from build123d import *

# Parameters (mm, degrees)
F1_DEPTH = 63.5
F0_W     = 25.755785
F0_H     = 19.05
F2_DEPTH = 25.4
F3_DEPTH = 7.9375
F4_R     = 6.35


with BuildPart() as f1:
    # F0 (on Front) → F1 (new body, symmetric)
    with BuildSketch(Plane.XZ):
        Polygon((41.275, -9.525), (41.275, 9.525), (22.225, 9.525), (-41.275, 9.525), (-41.275, -9.525), align=None)
    extrude(amount=F1_DEPTH, both=True)

    # F0 (on Front) → F2 (join, symmetric)
    with BuildSketch(Plane.XZ):
        with BuildLine():
            Line((22.225, 9.525), (41.275, 9.525))
            Line((41.275, 9.525), (41.275, 34.925))
            ThreePointArc((41.275, 34.925), (45.92468, 46.15032), (57.15, 50.8))
            Line((57.15, 50.8), (60.325, 50.8))
            Line((60.325, 50.8), (60.325, 69.85))
            Line((60.325, 69.85), (57.15, 69.85))
            ThreePointArc((57.15, 69.85), (32.454296, 59.620704), (22.225, 34.925))
            Line((22.225, 34.925), (22.225, 9.525))
        make_face()
        with Locations((73.202892, 60.325)):
            Rectangle(F0_W, F0_H)
    extrude(amount=F2_DEPTH, both=True)

    # F0 (on Front) → F3 (join, symmetric)
    with BuildSketch(Plane.XZ):
        with BuildLine():
            Line((-41.275, 9.525), (22.225, 9.525))
            Line((22.225, 9.525), (22.225, 34.925))
            ThreePointArc((22.225, 34.925), (32.454296, 59.620704), (57.15, 69.85))
            add(Edge.make_bspline(
                [(-41.275, 9.525), (-27.324263, 47.769934), (18.911634, 71.788173), (57.15, 69.85)],
                knots=[0, 0, 0, 0, 115.440834, 115.440834, 115.440834, 115.440834], degree=3))
        make_face()
    extrude(amount=F3_DEPTH, both=True)

    # F4
    f4_edges = [f1.edges().sort_by_distance(p)[0] for p in [
        (41.275, -63.5, 0),
        (-41.275, -63.5, 0),
        (41.275, 63.5, 0),
        (-41.275, 63.5, 0),
    ]]
    fillet(f4_edges, radius=F4_R)


solid = f1.part
Could you check a few things on this model? Use its own coordinates, in mm. A direction names the side the tool comes from. Give positions to 0.01 mm unless a question says otherwise; leave off trailing zeros. Order: outer loops, then holes, each group sorted by start corner. A loop starts at its lowest first (then second) coordinate and runs counter-clockwise, first axis right, second up.
1. Will these pins go through, and if not, where does the flat tip stop? P1, Ø16.5, axis at x = -8, y = -49.5, coming from the +Z side (3 decimals); P2, Ø22, axis at y = -28, z = 15, coming from the +X side (3 decimals); P3, Ø14.5, axis at x = 70.5, y = -5, coming from the -Z side.
2. For faces 1 (the cylindrical face through (32.727, -16.791, 59.891)), 2 (the flat face through (47, -25.4, 54)), 3 (the cylindrical face through (32.727, 16.547, 59.891)), 4 (the flat face through (71, 0, 50.8)), which set-ups out of +Z, -Z, +X, -X, +Y, -Y let a thin tool reach every point of the face, with its end or its side?
3. Suppose I cut it at B-B (y = -34). List the corners of the cut face in (x, z) for me (3 decimals), plus the area to 3 significant figures.
4. Suppose I cut it at A-A (z = 2.5). List the corners of the cut face in (x, y) for me (3 decimals).
5. I need wall thicknesses on L1, parallel to Z at x = 78, y = 17; L2, parallel to Z at x = 40, y = -44 (3 decimals); L3, parallel to X at y = 32, z = -3 (3 decimals). Which ranges of each line are inside material? Lowest first, please.
Solved:
1. P1: stops at z = 9.525
1. P2: stops at x = 41.275
1. P3: stops at z = 50.8
2. face 1: +Z, -X, -Y
2. face 2: +Z, +X, -X, -Y
2. face 3: +Z, -X, +Y
2. face 4: -Z, +X, +Y, -Y
3. outline: (-41.275, -9.525) - (41.275, -9.525) - (41.275, 9.525) - (-41.275, 9.525) - close
3. area: 1,570 mm2
4. outline: (-41.275, -57.15) arc R6.35 ccw to (-34.925, -63.5) - (34.925, -63.5) arc R6.35 ccw to (41.275, -57.15) - (41.275, 57.15) arc R6.35 ccw to (34.925, 63.5) - (-34.925, 63.5) arc R6.35 ccw to (-41.275, 57.15) - close
5. L1: z = 50.8 to 69.85
5. L2: z = -9.525 to 9.525
5. L3: x = -41.275 to 41.275
